Work out the finished part from the listing and answer in its coordinate system (mm). Face numbers are marked on the shaded views. A direction names the side the tool comes from. Round coordinates to 2 decimals unless told otherwise and drop trailing zeros. Write each loop counter-clockwise with the first axis right and the second up, starting at its lowest first coordinate (ties: lowest second). Pieces come first, ordered by that corner, then holes. Notation, with made-up numbers: (10.5, -35) -> (62.5, -35) arc R20 cw to (62.5, -29) -> close; hole circle Ø2 at (-33.5, 86). An arc over 180 degrees is marked (long way). Answer as a JSON object with one key per item and string values. Group by question number.
from build123d import *

# Parameters (mm, degrees)
CUT_EXTRUDE3_DEPTH = 22.225
SKETCH4_R          = 3.175
CUT_EXTRUDE4_DEPTH = 3.175


with BuildPart() as part:
    # Sketch2 → Revolve1 (revolve)
    with BuildSketch(Plane.XY):
        Polygon((6.35, 0), (6.35, 6.35), (3.175, 6.35), (3.175, 28.575), (1.5875, 28.575), (1.5875, 3.175), (3.175, 3.175), (3.175, 0), align=None)
    revolve(axis=Axis((0, 41.227012609, 0), (0, -1, 0)))

    # Sketch3 → Cut-Extrude3 (cut)
    with BuildSketch(Plane(origin=(0, 28.575, 0), x_dir=(1, 0, 0), z_dir=(0, 1, 0))):
        with BuildLine():
            Line((-3.175, 0), (-1.5875, 2.749630657))
            ThreePointArc((-1.5875, 2.749630657), (-2.749630657, 1.5875), (-3.175, 0))
        make_face()
        with BuildLine():
            ThreePointArc((1.5875, 2.749630657), (0, 3.175), (-1.5875, 2.749630657))
            Line((-1.5875, 2.749630657), (1.5875, 2.749630657))
        make_face()
        with BuildLine():
            ThreePointArc((3.175, 0), (2.749630657, 1.5875), (1.5875, 2.749630657))
            Line((1.5875, 2.749630657), (3.175, 0))
        make_face()
        with BuildLine():
            ThreePointArc((1.5875, -2.749630657), (2.749630657, -1.5875), (3.175, 0))
            Line((3.175, 0), (1.5875, -2.749630657))
        make_face()
        with BuildLine():
            Line((1.5875, -2.749630657), (-1.5875, -2.749630657))
            ThreePointArc((-1.5875, -2.749630657), (0, -3.175), (1.5875, -2.749630657))
        make_face()
        with BuildLine():
            Line((-1.5875, -2.749630657), (-3.175, 0))
            ThreePointArc((-3.175, 0), (-2.749630657, -1.5875), (-1.5875, -2.749630657))
        make_face()
    extrude(amount=-CUT_EXTRUDE3_DEPTH, mode=Mode.SUBTRACT)

    # Sketch4 → Cut-Extrude4 (cut)
    with BuildSketch(Plane.XZ):
        with BuildLine():
            ThreePointArc((-2.74963064, 1.58750003), (-1.587499985, 2.749630666), (0, 3.175))
            Line((0, 3.175), (-1.833087105, 3.175))
            Line((-1.833087105, 3.175), (-2.74963064, 1.58750003))
        make_face()
        with BuildLine():
            Line((2.749630611, 1.58750008), (1.833087105, 3.175))
            Line((1.833087105, 3.175), (0, 3.175))
            ThreePointArc((0, 3.175), (1.58749996, 2.74963068), (2.749630611, 1.58750008))
        make_face()
        with BuildLine():
            Line((3.666174209, 0), (2.749630611, 1.58750008))
            ThreePointArc((2.749630611, 1.58750008), (3.066814486, 0.821750513), (3.175, 0))
            ThreePointArc((3.175, 0), (3.066814483, -0.821750528), (2.749630596, -1.587500106))
            Line((2.749630596, -1.587500106), (3.666174209, 0))
        make_face()
        with BuildLine():
            Line((1.833087105, -3.175), (2.749630596, -1.587500106))
            ThreePointArc((2.749630596, -1.587500106), (1.587499947, -2.749630688), (0, -3.175))
            Line((0, -3.175), (1.833087105, -3.175))
        make_face()
        with BuildLine():
            ThreePointArc((0, -3.175), (-1.587499999, -2.749630657), (-2.749630656, -1.587500001))
            Line((-2.749630656, -1.587500001), (-1.833087105, -3.175))
            Line((-1.833087105, -3.175), (0, -3.175))
        make_face()
        with BuildLine():
            ThreePointArc((-2.749630656, -1.587500001), (-3.175, 1.7e-08), (-2.74963064, 1.58750003))
            Line((-2.74963064, 1.58750003), (-3.666174209, 0))
            Line((-3.666174209, 0), (-2.749630656, -1.587500001))
        make_face()
        Circle(SKETCH4_R)
    extrude(amount=-CUT_EXTRUDE4_DEPTH, mode=Mode.SUBTRACT)


solid = part.part
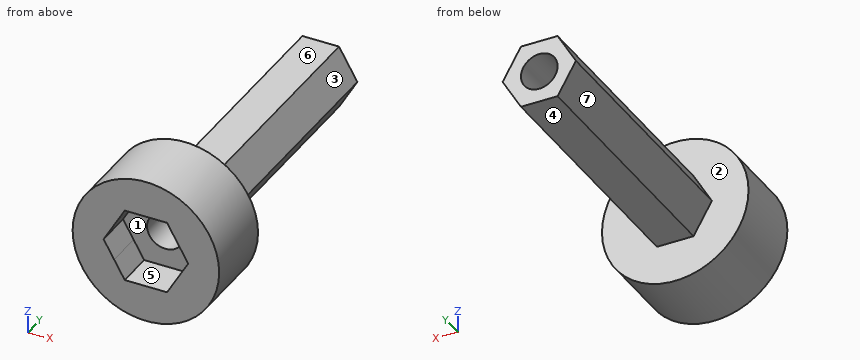
1) Straight lines are drawn through the part: L1, parallel to Z at x = 0, y = 19; L2, parallel to Y at x = -0.75, z = 3.25. For each, find the intervals that lie inside material, in ascending order.
2) For a pull along X with two mould halves and no side action, classify the marked faces 5, 6 and 7 as released by +X, released by -X, zero draft, split by the parting line, or undercut.
3) Each of these flat-tipped pins is pushed along its axis until it touches: P1, Ø1.6, axis at x = -0.5, y = 16, coming from the +Z side; P2, Ø1, axis at x = -3, y = 16.5, coming from the -Z side; P3, Ø4, axis at y = 17.5, z = 3, coming from the -X side. Where does it stop, or does it pass through?
4) A cutting plane is placed at C-C on z = 5. Determine the outline of the cut face in (x, y).
5) A tool of negligible diameter and unlimited length cuts with its end or side. For the marked faces 1, 2, 3 and 4, from which of +Z, -Z, +X, -X, +Y, -Y can it reach the whole face along a straight path? Write none if from no direction.
6) A cutting plane is placed at B-B on y = 16. Determine the outline of the cut face in (x, z) (1 decimal).
Established:
{
 "1": {"L1": "z = -2.75 to -1.59, 1.59 to 2.75", "L2": "y = 0 to 6.35"},
 "2": {"face 5": "undercut", "face 6": "zero draft", "face 7": "released by -X"},
 "3": {"P1": "stops at z = 2.75", "P2": "stops at z = -1.17", "P3": "stops at x = -2.6"},
 "4": {"outline": "(-3.91, 0) -> (3.91, 0) -> (3.91, 6.35) -> (-3.91, 6.35) -> close"},
 "5": {"face 1": "-Y", "face 2": "+Y", "face 3": "+Z, +X, +Y", "face 4": "-Z, +X, -X, +Y"},
 "6": {"outline": "(-3.2, 0) -> (-1.6, -2.7) -> (1.6, -2.7) -> (3.2, 0) -> (1.6, 2.7) -> (-1.6, 2.7) -> close; hole circle Ø3.2 at (0, 0)"}
}
